from build123d import *

# Parameters (mm, degrees)
F0_W     = 246
F0_H     = 454
F1_DEPTH = 12
F2_SIZE  = 11.99999
F4_D     = 3.5


# Not quite as in the source:
# - a fillet or chamfer is up to 0.001 mm smaller than in the source, because OpenCascade refuses the exact size


with BuildPart() as f1:
    # F0 (on Front) → F1 (new body)
    with BuildSketch(Plane.XZ):
        Rectangle(F0_W, F0_H)
    extrude(amount=F1_DEPTH)

    # F2 (size 12 in the source; OpenCascade refuses exactly that, so slightly less here)
    f2_edges = [f1.edges().sort_by_distance(p)[0] for p in [
        (0, 0, 227),
        (-123, 0, 0),
        (0, 0, -227),
        (123, 0, 0),
    ]]
    chamfer(f2_edges, length=F2_SIZE)

    # F4 (through all)
    with Locations(Plane.XZ.offset(12)):
        with Locations((-90.5, 207.5), (90.5, 207.5), (90.5, -207.5), (-90.5, -207.5)):
            Hole(F4_D / 2)


solid = f1.part
Input: part model. Units: mm. Frame: model coordinates. Give positions to 0.01 mm unless a question says otherwise; leave off trailing zeros. Write each loop counter-clockwise with the first axis right and the second up, starting at its lowest first coordinate (ties: lowest second). Pieces come first, ordered by that corner, then holes.
Q1. Section A-A, the plane y = -6. Output: boundary loops of the cut face in (x, z), plus the area to 3 significant figures.
Q2. First-contact query: P1, Ø1, axis at x = -95.5, y = -10, coming from the -Z side; P2, Ø1, axis at x = -17.5, y = -5, coming from the +Z side; P3, Ø2, axis at x = 51, y = -2, coming from the +Z side. Flat tips, straight axial feed; report the tip coordinate or a pass-through.
Q3. Material intervals for probe 1 along Z at (x, y) = (-90.5, -5); probe 2 along Z at (x, y) = (90.5, -7.5); probe 3 along X at (y, z) = (-4.25, -207.5), sorted ascending.
Q4. Pull-direction query (Y, two-part tool) for faces 1 (the face through (-2, -6, -221)), 2 (the face through (-2, -12, 3)); classes: pulls with the +Y half, pulls with the -Y half, needs draft (parallel to the pull), parting line crosses it, or undercut.
Filled in:
1. outline: (-117, -221) - (117, -221) - (117, 221) - (-117, 221) - close; hole circle Ø3.5 at (-90.5, -207.5); hole circle Ø3.5 at (-90.5, 207.5); hole circle Ø3.5 at (90.5, -207.5); hole circle Ø3.5 at (90.5, 207.5)
1. area: 103,000 mm2
2. P1: stops at z = -225.5
2. P2: stops at z = 220.5
2. P3: stops at z = 218
3. probe 1: z = -220 to -209.25, -205.75 to 205.75, 209.25 to 220
3. probe 2: z = -222.5 to -209.25, -205.75 to 205.75, 209.25 to 222.5
3. probe 3: x = -115.25 to -92.25, -88.75 to 88.75, 92.25 to 115.25
4. face 1: pulls with the +Y half
4. face 2: pulls with the -Y half
